Check sheet for the modelled part. Datum: model origin and axes. Units: mm. Face numbers are marked on the shaded views. A direction names the side the tool comes from. Coordinates: 2 decimals unless noted, no trailing zeros. Loops run counter-clockwise (first coordinate to the right, second up) from the corner with the lowest first, then second, coordinate; pieces in that order, holes last. Notation, with made-up numbers: M -18,-3 L 3,-3 A19 ccw 3,7 Z; hole C 38.5,72 d11. An arc over 180 degrees is marked long. Return JSON: item names as keys, results as strings.
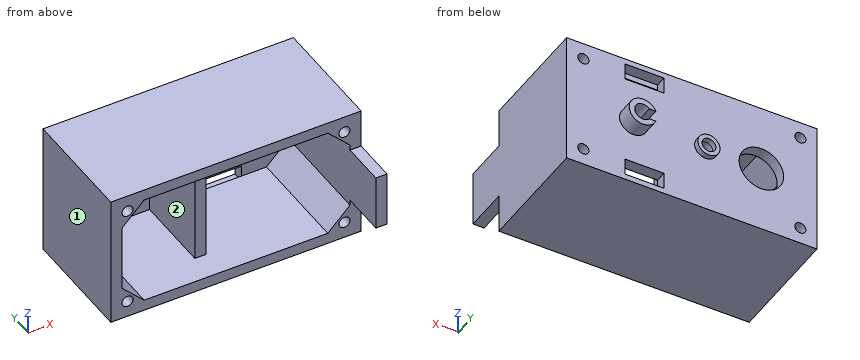
from build123d import *

# Parameters (mm, degrees)
SKETCH1_W           = 22.5
SKETCH1_H           = 12
SKETCH1_W_2         = 11.5
SKETCH1_H_2         = 10
SKETCH1_W_3         = 8
BOSS_EXTRUDE1_DEPTH = 10.5
SKETCH2_W           = 22.5
SKETCH2_H           = 12
SKETCH2_R           = 2
SKETCH2_R_2         = 0.75
SKETCH2_W_2         = 3.5
SKETCH2_H_2         = 1.5
BOSS_EXTRUDE2_DEPTH = 1
SKETCH3_W           = 3.5
SKETCH3_H           = 1.5
CUT_EXTRUDE1_DEPTH  = 1
SKETCH4_W           = 10
SKETCH4_H           = 2.5
CUT_EXTRUDE2_DEPTH  = 1
CHAMFER1_SIZE       = 2
SKETCH5_R           = 0.5
CUT_EXTRUDE3_DEPTH  = 11.5
SKETCH6_W           = 1
SKETCH6_H           = 5
BOSS_EXTRUDE3_DEPTH = 4
SKETCH7_R           = 1
SKETCH7_R_2         = 0.625
BOSS_EXTRUDE4_DEPTH = 1.75
SKETCH8_R           = 0.625
CUT_EXTRUDE4_DEPTH  = 1.75
SKETCH9_R           = 1
BOSS_EXTRUDE5_DEPTH = 0.25
SKETCH10_R          = 1
SKETCH10_R_2        = 0.625
BOSS_EXTRUDE6_DEPTH = 0.5
SKETCH11_R          = 1.25
SKETCH11_R_2        = 0.75
BOSS_EXTRUDE7_DEPTH = 1.5
CUT_EXTRUDE5_DEPTH  = 1.5


with BuildPart() as part:
    # Sketch1 → Boss-Extrude1 (new body)
    with BuildSketch(Plane(origin=(0, 0, 0), x_dir=(1, 0, 0), z_dir=(0, 1, 0))):
        Rectangle(SKETCH1_W, SKETCH1_H)
        with Locations((4.5, 0)):
            Rectangle(SKETCH1_W_2, SKETCH1_H_2, mode=Mode.SUBTRACT)
        with Locations((-6.25, 0)):
            Rectangle(SKETCH1_W_3, SKETCH1_H_2, mode=Mode.SUBTRACT)
    extrude(amount=BOSS_EXTRUDE1_DEPTH)

    # Sketch2 → Boss-Extrude2 (add)
    with BuildSketch(Plane(origin=(0, 10.5, 0), x_dir=(1, 0, 0), z_dir=(0, 1, 0))):
        Rectangle(SKETCH2_W, SKETCH2_H)
        with Locations((-6.25, 0)):
            Circle(SKETCH2_R, mode=Mode.SUBTRACT)
        with Locations((5.25, 0)):
            Circle(SKETCH2_R_2, mode=Mode.SUBTRACT)
        with Locations((4.25, 4.75)):
            Rectangle(SKETCH2_W_2, SKETCH2_H_2, mode=Mode.SUBTRACT)
        with Locations((4.25, -4.75)):
            Rectangle(SKETCH2_W_2, SKETCH2_H_2, mode=Mode.SUBTRACT)
    extrude(amount=-BOSS_EXTRUDE2_DEPTH)

    # Sketch3 → Cut-Extrude1 (cut)
    with BuildSketch(Plane(origin=(0, 10.5, 0), x_dir=(1, 0, 0), z_dir=(0, 1, 0))):
        with Locations((4.25, 4.75)):
            Rectangle(SKETCH3_W, SKETCH3_H)
        with Locations((4.25, -4.75)):
            Rectangle(SKETCH3_W, SKETCH3_H)
    extrude(amount=-CUT_EXTRUDE1_DEPTH, mode=Mode.SUBTRACT)

    # Sketch4 → Cut-Extrude2 (cut)
    with BuildSketch(Plane.ZY.offset(2.25)):
        with Locations((0, 1.25)):
            Rectangle(SKETCH4_W, SKETCH4_H)
    extrude(amount=-CUT_EXTRUDE2_DEPTH, mode=Mode.SUBTRACT)

    # Chamfer1
    chamfer1_edges = [part.edges().sort_by_distance(p)[0] for p in [
        (-10.25, 4.75, 5),
        (-10.25, 4.75, -5),
        (10.25, 4.75, -5),
        (10.25, 4.75, 5),
    ]]
    chamfer(chamfer1_edges, length=CHAMFER1_SIZE)

    # Sketch5 → Cut-Extrude3 (cut, through all)
    with BuildSketch(Plane.XZ):
        with Locations((-9.75, 4.5)):
            Circle(SKETCH5_R)
        with Locations((9.75, 4.5)):
            Circle(SKETCH5_R)
        with Locations((9.75, -4.5)):
            Circle(SKETCH5_R)
        with Locations((-9.75, -4.5)):
            Circle(SKETCH5_R)
    extrude(amount=-CUT_EXTRUDE3_DEPTH, mode=Mode.SUBTRACT)

    # Sketch6 → Boss-Extrude3 (add)
    with BuildSketch(Plane.XZ):
        with Locations((10.75, 0)):
            Rectangle(SKETCH6_W, SKETCH6_H)
    extrude(amount=BOSS_EXTRUDE3_DEPTH)

    # Sketch7 → Boss-Extrude4 (add)
    with BuildSketch(Plane(origin=(0, 10.5, 0), x_dir=(1, 0, 0), z_dir=(0, 1, 0))):
        with Locations((-1.25, 0)):
            Circle(SKETCH7_R)
        with Locations((-1.25, 0)):
            Circle(SKETCH7_R_2, mode=Mode.SUBTRACT)
    extrude(amount=-BOSS_EXTRUDE4_DEPTH)

    # Sketch8 → Cut-Extrude4 (cut)
    with BuildSketch(Plane(origin=(0, 10.5, 0), x_dir=(1, 0, 0), z_dir=(0, 1, 0))):
        with Locations((-1.25, 0)):
            Circle(SKETCH8_R)
    extrude(amount=-CUT_EXTRUDE4_DEPTH, mode=Mode.SUBTRACT)

    # Sketch9 → Boss-Extrude5 (add)
    with BuildSketch(Plane.XZ.offset(-8.75)):
        with Locations((-1.25, 0)):
            Circle(SKETCH9_R)
    extrude(amount=BOSS_EXTRUDE5_DEPTH)

    # Sketch10 → Boss-Extrude6 (add)
    with BuildSketch(Plane(origin=(0, 10.5, 0), x_dir=(1, 0, 0), z_dir=(0, 1, 0))):
        with Locations((-1.25, 0)):
            Circle(SKETCH10_R)
        with Locations((-1.25, 0)):
            Circle(SKETCH10_R_2, mode=Mode.SUBTRACT)
    extrude(amount=BOSS_EXTRUDE6_DEPTH)

    # Sketch11 → Boss-Extrude7 (add)
    with BuildSketch(Plane(origin=(0, 10.5, 0), x_dir=(1, 0, 0), z_dir=(0, 1, 0))):
        with Locations((5.25, 0)):
            Circle(SKETCH11_R)
        with Locations((5.25, 0)):
            Circle(SKETCH11_R_2, mode=Mode.SUBTRACT)
    extrude(amount=BOSS_EXTRUDE7_DEPTH)

    # Sketch12 → Cut-Extrude5 (cut)
    with BuildSketch(Plane(origin=(0, 12, 0), x_dir=(1, 0, 0), z_dir=(0, 1, 0))):
        with BuildLine():
            Line((4.104356076, 0.5), (4.690983006, 0.5))
            ThreePointArc((4.690983006, 0.5), (4.5, 0), (4.690983006, -0.5))
            Line((4.690983006, -0.5), (4.104356076, -0.5))
            ThreePointArc((4.104356076, -0.5), (4, 0), (4.104356076, 0.5))
        make_face()
    extrude(amount=-CUT_EXTRUDE5_DEPTH, mode=Mode.SUBTRACT)


solid = part.part
1) Set-up check for the marked faces 1 and 2: record each of +Z, -Z, +X, -X, +Y, -Y from which the full face is reachable in a straight line by a thin tool's end or side.
Answers:
{"face 1": "+Z, -Z, -X, +Y, -Y", "face 2": "-Y"}
2) Section check C-C on x = 5.25. Record the cut outline in (y, z), then the cut area to 3 significant figures.
Answers:
{"outline": "M 0,-6 L 10.5,-6 L 10.5,-5.5 L 9.5,-5.5 L 9.5,-5 L 0,-5 Z; M 0,5 L 9.5,5 L 9.5,5.5 L 10.5,5.5 L 10.5,6 L 0,6 Z; M 9.5,-4 L 10.5,-4 L 10.5,-1.25 L 12,-1.25 L 12,-0.75 L 9.5,-0.75 Z; M 9.5,0.75 L 12,0.75 L 12,1.25 L 10.5,1.25 L 10.5,4 L 9.5,4 Z", "area": "28.0 mm²"}
3) Go/stop test with flat-tipped pins: pin 1 Ø2 at (x, z) = (6.5, 3.5) entering from +Y; pin 2 Ø6 at (x, z) = (2.5, -3.5) entering from -Y; pin 3 Ø0.6 at (x, y) = (4.5, 11.5) entering from -Z. Record where each tip stops, or that it passes through.
Answers:
{"pin 1": "y = 10.5", "pin 2": "y = 0", "pin 3": "z = -1.17"}
4) Section check D-D on z = 0. Count the separate pieces of the cut face and the enclosed holes in it, then the cut area to 3 significant figures.
Answers:
{"separate pieces": "3", "enclosed holes": "0", "area": "46.9 mm²"}
5) Section check B-B on z = -4.5. Record the cut outline in (x, y).
Answers:
{"outline": "M -11.25,0 L -10.25,0 L -10.25,10.5 L -11.25,10.5 Z; M -9.25,0 L -8.75,0 L -8.75,9.5 L -2.25,9.5 L -2.25,2.5 L -1.25,2.5 L -1.25,9.5 L 2.5,9.5 L 2.5,10.5 L -9.25,10.5 Z; M 6,9.5 L 8.75,9.5 L 8.75,0 L 9.25,0 L 9.25,10.5 L 6,10.5 Z; M 10.25,0 L 11.25,0 L 11.25,10.5 L 10.25,10.5 Z"}
6) Scan lines: line 1 along X through (y, z) = (10.7, 0) (3 decimals); line 2 along X through (y, z) = (9.95, 0) (3 decimals); line 3 along Z through (x, y) = (-3.5, 7.5). Record each from-to range of solid material in increasing order. Write a range as [from, to].
Answers:
{"line 1": "[-2.25, -1.875], [-0.625, -0.25], [6, 6.5]", "line 2": "[-11.25, -8.25], [-4.25, -1.875], [-0.625, 4.5], [6, 11.25]", "line 3": "[-6, -5], [5, 6]"}
7) Section check A-A on x = 9.75. Record the cut outline in (y, z).
Answers:
{"outline": "M 0,-6 L 10.5,-6 L 10.5,-5 L 0,-5 Z; M 0,-4 L 10.5,-4 L 10.5,4 L 0,4 L 0,3.5 L 9.5,3.5 L 9.5,-3.5 L 0,-3.5 Z; M 0,5 L 10.5,5 L 10.5,6 L 0,6 Z"}
